Check sheet for the modelled part. Datum: model origin and axes. Units: mm. A direction names the side the tool comes from. Coordinates: 2 decimals unless noted, no trailing zeros. Loops run counter-clockwise (first coordinate to the right, second up) from the corner with the lowest first, then second, coordinate; pieces in that order, holes last. Notation, with made-up numbers: (-6, 39.25) - (47, 39.25) arc R11 ccw to (47, 50.25) - close; hole circle Ø10 at (34, -36). An arc over 180 degrees is marked (long way). Use a Markdown table: item, result. Add a question column.
1) Sectioned sample at B-B, the plane x = -10.75. Enter the section's corners in (y, z).
2) Sectioned sample at C-C, the plane y = 3. Enter the section's corners in (x, z), then the cut area to 3 significant figures.
3) Draft check along Y on faces 5 (the flat face through (-1.184, 3.075, -93.916)), 6 (the flat face through (-3, 19.17, -94)), 7 (the flat face through (-9, 7, -190.5)). Enter one of: pulls with the +Y half, pulls with the -Y half, needs draft (parallel to the pull), parting line crosses it, or undercut.
4) Go/stop test with flat-tipped pins: P1, Ø6, axis at y = 12.5, z = -35.5, coming from the -X side; P2, Ø3, axis at y = 16.5, z = -28, coming from the -X side; P3, Ø10, axis at x = -15.5, z = -59.5, coming from the -Y side; P4, Ø1, axis at y = 14.5, z = -142, coming from the +X side. Record where each tip stops, or that it passes through.
5) Sectioned sample at A-A, the plane z = -98. Enter the section's corners in (x, y).
6) Thickness scan on line 1 (Y direction, x = -2.5, z = -129); line 2 (X direction, y = 8.5, z = -59); line 3 (X direction, y = 17.5, z = -92). Record the ranges inside material, lowest first.
7) Tool access check on faces 1 (the flat face through (-11.15, 14.9, -93.92)), 2 (the flat face through (-3, 20.186, -94)), 3 (the flat face through (-0.175, 3.219, -93.916)), 4 (the flat face through (-10, 6.295, -94)). Record the directions out of +Z, -Z, +X, -X, +Y, -Y that give a thin tool (end or side, any length) a straight path to the whole face; none if there is none.
from build123d import *

# Parameters (mm, degrees)
BOSS_EXTRUDE1_DEPTH = 190.5
FILLET1_R           = 1.016


with BuildPart() as part:
    # Sketch1 → Boss-Extrude1 (new body)
    with BuildSketch(Plane.XY):
        with BuildLine():
            Line((-1.014506285, -0.055072655), (-1.359217172, 6.294927345))
            Line((-1.359217172, 6.294927345), (-19.05, 6.294927345))
            Line((-19.05, 6.294927345), (-19.05, 11.057427345))
            Line((-19.05, 11.057427345), (-4.7625, 20.185552345))
            Line((-4.7625, 20.185552345), (-1.016, 20.185552345))
            ThreePointArc((-1.016, 20.185552345), (-0.212054439, 19.790783006), (-0.032858991, 18.913252215))
            Line((-0.032858991, 18.913252215), (-0.79375, 15.994552345))
            Line((-0.79375, 15.994552345), (-1.776891009, 16.250852474))
            Line((-1.776891009, 16.250852474), (-1.016, 19.169552345))
            Line((-1.016, 19.169552345), (-4.465650477, 19.169552345))
            Line((-4.465650477, 19.169552345), (-18.034, 10.500884594))
            Line((-18.034, 10.500884594), (-18.034, 7.310927345))
            Line((-18.034, 7.310927345), (-0.396875, 7.310927345))
            Line((-0.396875, 7.310927345), (0, 0))
            Line((0, 0), (-1.014506285, -0.055072655))
        make_face()
    extrude(amount=-BOSS_EXTRUDE1_DEPTH)

    # Fillet1
    fillet1_edges = [part.edges().sort_by_distance(p)[0] for p in [
        (-19.05, 6.294927345, -95.25),
        (-19.05, 11.057427345, -95.25),
        (-4.7625, 20.185552345, -95.25),
        (-0.396875, 7.310927345, -95.25),
    ]]
    fillet(fillet1_edges, radius=FILLET1_R)


solid = part.part
Solved:
| question | item | result |
|---|---|---|
| 1 | outline | (6.29, -190.5) - (7.31, -190.5) - (7.31, 0) - (6.29, 0) - close; (15.15, -190.5) - (16.36, -190.5) - (16.36, 0) - (15.15, 0) - close |
| 2 | outline | (-1.18, -190.5) - (-0.16, -190.5) - (-0.16, 0) - (-1.18, 0) - close |
| 2 | area | 194 mm2 |
| 3 | face 5 | pulls with the -Y half |
| 3 | face 6 | undercut |
| 3 | face 7 | needs draft |
| 4 | P1 | stops at x = -19.05 |
| 4 | P2 | stops at x = -12.88 |
| 4 | P3 | stops at y = 6.29 |
| 4 | P4 | stops at x = -10.99 |
| 5 | outline | (-19.05, 7.31) arc R1.02 ccw to (-18.03, 6.29) - (-1.36, 6.29) - (-1.01, -0.06) - (0, 0) - (-0.34, 6.35) arc R1.02 ccw to (-1.36, 7.31) - (-18.03, 7.31) - (-18.03, 10.5) - (-4.47, 19.17) - (-1.02, 19.17) - (-1.78, 16.25) - (-0.79, 15.99) - (-0.03, 18.91) arc R1.02 ccw to (-1.02, 20.19) - (-4.47, 20.19) arc R1.02 ccw to (-5.01, 20.03) - (-18.58, 11.36) arc R1.02 ccw to (-19.05, 10.5) - close |
| 6 | line 1 | y = 6.29 to 7.31, 19.17 to 20.19 |
| 6 | line 2 | x = -19.05 to -18.03 |
| 6 | line 3 | x = -8.97 to -7.08, -1.45 to -0.4 |
| 7 | face 1 | +Z, -Z |
| 7 | face 2 | +Z, -Z, +X, -X, +Y |
| 7 | face 3 | +Z, -Z, +X |
| 7 | face 4 | +Z, -Z, -X, -Y |
